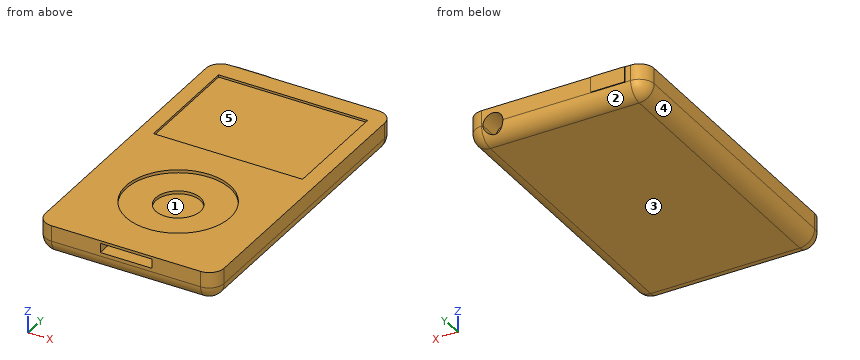
from build123d import *

# Parameters (mm, degrees)
F0_R      = 17.78
F0_W      = 50.8
F0_H      = 38.1
F1_DEPTH  = 10.414
F2_DEPTH  = 9.652
F0_R_2    = 7.62
F3_DEPTH  = 9.398
F4_DEPTH  = 8.382
F5_R      = 5.08
F6_W      = 17.5757724792
F6_H      = 3.1867753714
F7_DEPTH  = 7.874
F8_W      = 11.499017477
F8_H      = 5.2686166653
F9_DEPTH  = 0.254
F10_DEPTH = 7.62


with BuildPart() as f1:
    # F0 (on Top) → F1 (new body)
    with BuildSketch(Plane.XY):
        with BuildLine():
            Line((25.4, 52.07), (-25.4, 52.07))
            ThreePointArc((-25.4, 52.07), (-28.9921024484, 50.5821024484), (-30.48, 46.99))
            Line((-30.48, 46.99), (-30.48, -46.99))
            ThreePointArc((-30.48, -46.99), (-28.9921024484, -50.5821024484), (-25.4, -52.07))
            Line((-25.4, -52.07), (25.4, -52.07))
            ThreePointArc((25.4, -52.07), (28.9921024484, -50.5821024484), (30.48, -46.99))
            Line((30.48, -46.99), (30.48, 46.99))
            ThreePointArc((30.48, 46.99), (28.9921024484, 50.5821024484), (25.4, 52.07))
        make_face()
        with Locations((0, -21.59)):
            Circle(F0_R, mode=Mode.SUBTRACT)
        with Locations((0, 26.67)):
            Rectangle(F0_W, F0_H, mode=Mode.SUBTRACT)
    extrude(amount=F1_DEPTH)

    # F0 (on Top) → F2 (join)
    with BuildSketch(Plane.XY):
        with Locations((0, 26.67)):
            Rectangle(F0_W, F0_H)
    extrude(amount=F2_DEPTH)

    # F0 (on Top) → F3 (join)
    with BuildSketch(Plane.XY):
        with Locations((0, -21.59)):
            Circle(F0_R)
        with Locations((0, -21.59)):
            Circle(F0_R_2, mode=Mode.SUBTRACT)
    extrude(amount=F3_DEPTH)

    # F0 (on Top) → F4 (join)
    with BuildSketch(Plane.XY):
        with Locations((0, -21.59)):
            Circle(F0_R_2)
    extrude(amount=F4_DEPTH)

    # F5
    f5_edges = [f1.edges().sort_by_distance(p)[0] for p in [
        (-28.992102, -50.582102, 0),
    ]]
    fillet(f5_edges, radius=F5_R)

    # F6 (on face) → F7 (cut)
    with BuildSketch(Plane.XZ.offset(52.07)):
        with Locations((0, 7.9176947474)):
            Rectangle(F6_W, F6_H)
    extrude(amount=-F7_DEPTH, mode=Mode.SUBTRACT)

    # F8 (on face) → F9 (join)
    with BuildSketch(Plane(origin=(0, 52.07, 0), x_dir=(-1, 0, 0), z_dir=(0, 1, 0))):
        with Locations((17.6987573504, 7.7143083327)):
            Rectangle(F8_W, F8_H)
    extrude(amount=F9_DEPTH)

    # F8 (on face) → F10 (cut)
    with BuildSketch(Plane(origin=(0, 52.07, 0), x_dir=(-1, 0, 0), z_dir=(0, 1, 0))):
        with BuildLine():
            ThreePointArc((-24.9499100409, 5.08), (-21.5465091169, 1.676599076), (-18.1431081928, 5.08))
            Line((-18.1431081928, 5.08), (-24.9499100409, 5.08))
        make_face()
        with BuildLine():
            Line((-24.9499100409, 5.08), (-18.1431081928, 5.08))
            ThreePointArc((-18.1431081928, 5.08), (-21.5465091169, 8.483400924), (-24.9499100409, 5.08))
        make_face()
    extrude(amount=-F10_DEPTH, mode=Mode.SUBTRACT)


solid = f1.part
Design review of the part built by this model. Coordinates are the model's own, in mm. Face numbers are marked on the shaded views. A direction names the side the tool comes from. Coordinates: 2 decimals unless noted, no trailing zeros. Write each loop counter-clockwise with the first axis right and the second up, starting at its lowest first coordinate (ties: lowest second). Pieces come first, ordered by that corner, then holes. Notation, with made-up numbers: (80, -30.5) -> (105, -30.5) arc R22 cw to (105, 7.5) -> close; hole circle Ø1 at (88.5, 11.25). An arc over 180 degrees is marked (long way). Write each question's results on one line, items separated by ' | '. Start each with the question number.
(1) For line 1 along Y through (x, z) = (0, 9.15); line 2 along Y through (x, z) = (0, 9.9); line 3 along Z through (x, y) = (-1, -34), list the stretches that pass through material, from the lowest coordinate up. Write a range as from..to.
(2) Tool access review of the marked faces 1 and 2: name each direction out of +Z, -Z, +X, -X, +Y, -Y from which nothing blocks a thin tool from reaching the whole face with its end or side.
(3) Take a section at D-D on y = -21.59. Write out the cut boundary in (x, z).
(4) The part is to be moulded in two halves that separate along X. For the marked faces 3, 4 and 5, say which applies: pulls with the +X half, pulls with the -X half, needs draft (parallel to the pull), parting line crosses it, or undercut.
(5) Clearance check with flat-ended pins moving along their axes: P1, Ø3.5, axis at x = 20, z = 5.5, coming from the +Y side; P2, Ø4, axis at x = -13, y = 35.5, coming from the +Z side; P3, Ø1, axis at y = -48.5, z = 8, coming from the +X side. State where each tip first meets the part, or that it passes through.
(6) Take a section at A-A on y = 39. Write out the cut boundary in (x, z).
(7) Take a section at C-C on z = 3. Write out the cut boundary in (x, y), and give its area (3 significant figures).
(8) Take a section at B-B on x = 0. Write out the cut boundary in (y, z), and give its area (3 significant figures).
Results found:
1) line 1: y = -44.2..-29.21, -13.97..52.07 | line 2: y = -52.07..-39.37, -3.81..7.62, 45.72..52.07 | line 3: z = 0..9.4
2) face 1: +Z | face 2: -Z, +X, -X, +Y
3) outline: (-30.48, 5.08) arc R5.08 ccw to (-25.4, 0) -> (25.4, 0) arc R5.08 ccw to (30.48, 5.08) -> (30.48, 10.41) -> (17.78, 10.41) -> (17.78, 9.4) -> (7.62, 9.4) -> (7.62, 8.38) -> (-7.62, 8.38) -> (-7.62, 9.4) -> (-17.78, 9.4) -> (-17.78, 10.41) -> (-30.48, 10.41) -> close
4) face 3: needs draft | face 4: pulls with the -X half | face 5: undercut
5) P1: stops at y = 44.45 | P2: stops at z = 9.65 | P3: stops at x = 30.38
6) outline: (-30.48, 5.08) arc R5.08 ccw to (-25.4, 0) -> (25.4, 0) arc R5.08 ccw to (30.48, 5.08) -> (30.48, 10.41) -> (25.4, 10.41) -> (25.4, 9.65) -> (-25.4, 9.65) -> (-25.4, 10.41) -> (-30.48, 10.41) -> close
7) outline: (-30.03, -46.99) arc R4.63 ccw to (-25.4, -51.62) -> (25.4, -51.62) arc R4.63 ccw to (30.03, -46.99) -> (30.03, 46.99) arc R4.63 ccw to (25.4, 51.62) -> (24.24, 51.62) -> (24.24, 44.45) -> (18.85, 44.45) -> (18.85, 51.62) -> (-25.4, 51.62) arc R4.63 ccw to (-30.03, 46.99) -> close | area: 6,150 mm2
8) outline: (-52.07, 5.08) arc R5.08 ccw to (-46.99, 0) -> (46.99, 0) arc R5.08 ccw to (52.07, 5.08) -> (52.07, 10.41) -> (45.72, 10.41) -> (45.72, 9.65) -> (7.62, 9.65) -> (7.62, 10.41) -> (-3.81, 10.41) -> (-3.81, 9.4) -> (-13.97, 9.4) -> (-13.97, 8.38) -> (-29.21, 8.38) -> (-29.21, 9.4) -> (-39.37, 9.4) -> (-39.37, 10.41) -> (-52.07, 10.41) -> (-52.07, 9.51) -> (-44.2, 9.51) -> (-44.2, 6.32) -> (-52.07, 6.32) -> close | area: 968 mm2
